CAD build for the part. Positions are in the model's coordinates, mm. Coordinates: 2 decimals unless noted, no trailing zeros. Loops run counter-clockwise (first coordinate to the right, second up) from the corner with the lowest first, then second, coordinate; pieces in that order, holes last.
1) Saw through at A-A, the plane z = 2.2. Give the number of separate pieces and of enclosed holes in the cut face, and give its area (3 significant figures).
2) Wall check: line 1 along X through (y, z) = (-86, 2.4); line 2 along X through (y, z) = (-33.5, 2); line 3 along Y through (x, z) = (12, 2.65). Give the ranges that are in metal, low to high.
3) Saw through at B-B, the plane x = 7. Write the cut outline in (y, z).
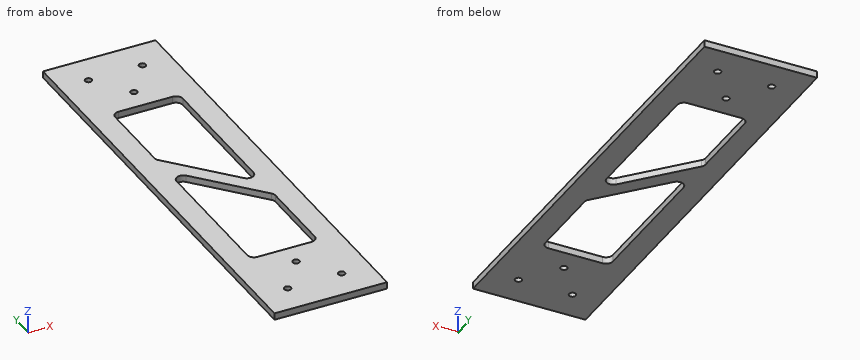
Autodesk Inventor part; units mm, degrees
ref_plane "YZ Plane" through (0, 0, 0) normal (1, 0, 0) x (0, 1, 0)
ref_plane "XZ Plane" through (0, 0, 0) normal (0, 1, 0) x (-1, 0, 0)
ref_plane "XY Plane" through (0, 0, 0) normal (0, 0, 1) x (1, 0, 0)
sketch "Szkic1" plane through (0, 0, 0) normal (0, 0, 1) x (1, 0, 0)
  line L0 (-25, -100) -> (25, -100)
  line L1 (25, -100) -> (25, 100)
  line L2 (25, 100) -> (-25, 100)
  line L3 (-25, 100) -> (-25, -100)
  line L4 (-25, -100) -> (25, 100) construction
  line L5 (25, -100) -> (-25, 100) construction
  point P0 (0, 0)
  dimension "d0" = 50
  dimension "d1" = 200
extrude "Wyciągnięcie proste1" add sketch "Szkic1" along normal blind 3
sketch "Szkic3" plane through (0, 0, 3) normal (0, 0, 1) x (1, 0, 0)
  line L0 (-25, -100) -> (25, -100)
  line L1 (25, 100) -> (-25, 100)
  line L2 (0, 100) -> (0, -100) construction
  line L3 (-25, 100) -> (-25, -100)
  line L4 (-25, 0) -> (25, 0) construction
  point P0 (0, 0)
  point P1 (-12, -86)
  point P2 (12, -86)
  point P3 (0, -70)
  point P4 (-12, 86)
  point P5 (12, 86)
  point P6 (0, 70)
  dimension "d21" = 14
  dimension "d22" = 14
  dimension "d23" = 24
  dimension "d24" = 12
  dimension "d25" = 30
hole "Otwór1" at (-12, -86, 3) at (12, -86, 3) at (0, -70, 3) at (0, 70, 3) at (12, 86, 3) at (-12, 86, 3) direction (0, 0, -1) diameter 3 depth 8 tip angle 118
sketch "Szkic4" plane through (0, 0, 3) normal (0, 0, 1) x (1, 0, 0)
  line L0 (-25, 100) -> (-25, -100)
  line L1 (25, -100) -> (25, 100)
  line L2 (15, -12) -> (0, 5)
  line L3 (-15, 60) -> (-15, 22)
  line L4 (0, 5) -> (-15, 22)
  line L5 (-15, 60) -> (15, 60)
  line L6 (25, -100) -> (25, 100)
  line L7 (15, 60) -> (15, -12)
  line L8 (-15, -60) -> (15, -60)
  line L9 (15, -60) -> (15, -22)
  line L10 (15, -22) -> (-15, 12)
  line L11 (-15, 12) -> (-15, -60)
  point P0 (0, 0)
  dimension "d33" = 10
  dimension "d34" = 10
  dimension "d35" = 60
  dimension "d36" = 60
  dimension "d37" = 5
  dimension "d38" = 25
  dimension "d39" = 10
  dimension "d40" = 12
  dimension "d41" = 10
  dimension "d42" = 10
  dimension "d43" = 10
  dimension "d44" = 10
  dimension "d45" = 60
  dimension "d46" = 60
extrude "Wyciągnięcie proste3" cut sketch "Szkic4" against normal blind 3
fillet "Zaokrąglenie1" radius 3 8 edges at (15, -12, 1.5) (-15, 22, 1.5) (15, 60, 1.5) (-15, 60, 1.5) (-15, 12, 1.5) (15, -22, 1.5) (-15, -60, 1.5) (15, -60, 1.5)
properties part number "Bok" material "Aluminium 6061"
Data:
1. separate pieces: 1
1. enclosed holes: 8
1. area: 6,690 mm2
2. line 1: x = -25 to -13.5, -10.5 to 10.5, 13.5 to 25
2. line 2: x = -25 to -15, 15 to 25
2. line 3: y = -100 to -87.5, -84.5 to -60, -18.6 to -7.07, 60 to 84.5, 87.5 to 100
3. outline: (-100, 0) - (-60, 0) - (-60, 3) - (-100, 3) - close; (-12.93, 0) - (-2.93, 0) - (-2.93, 3) - (-12.93, 3) - close; (60, 0) - (100, 0) - (100, 3) - (60, 3) - close
